The listing builds one solid part. Answer for the finished solid, in the listing's coordinates (mm). Face numbers are marked on the shaded views. Give positions to 0.01 mm unless a question says otherwise; leave off trailing zeros. Order: outer loops, then holes, each group sorted by start corner. A loop starts at its lowest first (then second) coordinate and runs counter-clockwise, first axis right, second up. Notation, with made-up numbers: (71, -14) - (113, -14) arc R11 cw to (113, -9) - close; hole circle Ø1 at (68.5, 37.25). An arc over 180 degrees is marked (long way). Answer in a Markdown table with one row per item. Add a question column.
```python
from build123d import *

# Parameters (mm, degrees)
SKETCH_R     = 45
PAD_DEPTH    = 160
FILLET_R     = 3
SKETCH001_R  = 40
POCKET_DEPTH = 150
FILLET001_R  = 1


with BuildPart() as part:
    # Sketch → Pad (new body)
    with BuildSketch(Plane.XY):
        Circle(SKETCH_R)
    extrude(amount=PAD_DEPTH)

    # Fillet
    fillet_edges = [part.edges().sort_by_distance(p)[0] for p in [
        (-45, 0, 160),
    ]]
    fillet(fillet_edges, radius=FILLET_R)

    # Sketch001 (on Face4 of Fillet) → Pocket (cut)
    with BuildSketch(Plane.XY.offset(160)):
        Circle(SKETCH001_R)
    extrude(amount=-POCKET_DEPTH, mode=Mode.SUBTRACT)

    # Fillet001
    fillet001_edges = [part.edges().sort_by_distance(p)[0] for p in [
        (-40, 0, 160),
    ]]
    fillet(fillet001_edges, radius=FILLET001_R)


solid = part.part
```
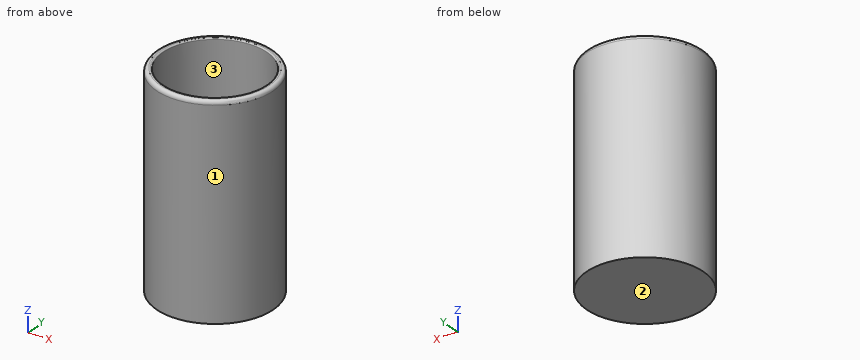
(1) Straight lines are drawn through the part: line 1 (Y direction, x = 0, z = 117.5); line 2 (Z direction, x = -4.5, y = 37.5); line 3 (Y direction, x = 16.5, z = 129). For each, find the intervals that lie inside material, in ascending order.
(2) Find section B-B, the plane z = 100. Write down the section's boundary in (x, y), plus the area to 3 significant figures.
(3) Each of these flat-tipped pins is pushed along its axis until it touches: P1, Ø10, axis at x = -1.5, z = 123, coming from the +Y side; P2, Ø6, axis at x = -32, z = 20.5, coming from the +Y side; P3, Ø5, axis at y = 7, z = 75.5, coming from the +X side; P4, Ø6, axis at x = -1.5, y = -30.5, coming from the -Z side. Where does it stop, or does it pass through?
(4) The mould has two halves that part along X. Classify the marked faces 1, 2 and 3: +X half, -X half, draft (parallel to the pull), parting line (faces both ways), or undercut.
(5) Find section A-A, the plane y = 0. Write down the section's boundary in (x, z).
Answer key:
| question | item | result |
|---|---|---|
| 1 | line 1 | -45 to -40, 40 to 45 |
| 1 | line 2 | 0 to 10 |
| 1 | line 3 | -41.87 to -36.44, 36.44 to 41.87 |
| 2 | outline | circle Ø90 at (0, 0); hole circle Ø80 at (0, 0) |
| 2 | area | 1,340 mm² |
| 3 | P1 | y = 45 |
| 3 | P2 | y = 34.41 |
| 3 | P3 | x = 44.77 |
| 3 | P4 | z = 0 |
| 4 | face 1 | parting line |
| 4 | face 2 | draft |
| 4 | face 3 | undercut |
| 5 | outline | (-45, 0) - (45, 0) - (45, 157) arc R3 ccw to (42, 160) - (41, 160) arc R1 ccw to (40, 159) - (40, 10) - (-40, 10) - (-40, 159) arc R1 ccw to (-41, 160) - (-42, 160) arc R3 ccw to (-45, 157) - close |
